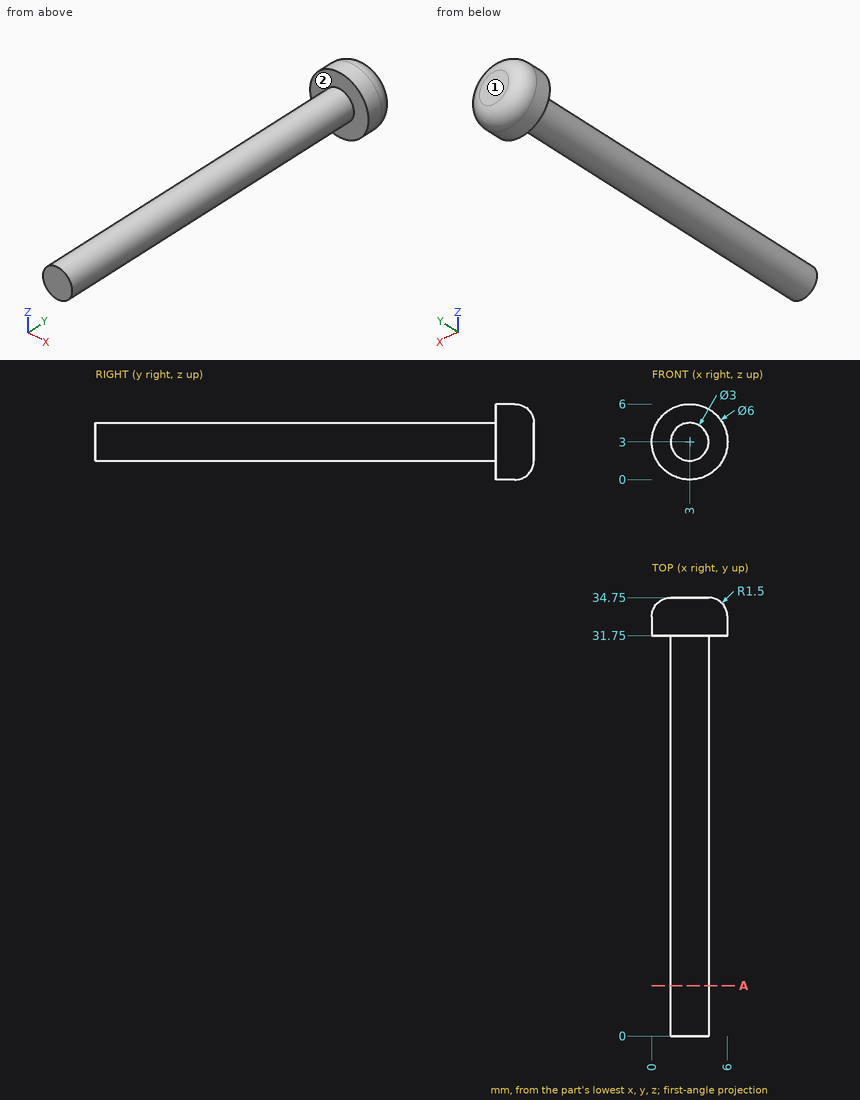
Job drawing, mm, ordinate dimensions from the low corner. One solid piece. A direction names the side the tool comes from. Coordinates: 2 decimals unless noted, no trailing zeros. Order: outer loops, then holes, each group sorted by start corner. A loop starts at its lowest first (then second) coordinate and runs counter-clockwise, first axis right, second up. Notation, with made-up numbers: (24, 35) - (30, 35) arc R23 cw to (30, 51) - close; hole circle Ø1 at (87.5, 53.5). An arc over 180 degrees is marked (long way). Write each question's results on one line, items separated by ' | '. Start each with the question number.
Item 1: Band-saw the part on A-A on y = 4. Write the cut outline in (x, z).
Item 2: Flat gauge pin, fed straight in: pin 1 (2 mm diameter, centred on x = 1, z = 3.5, fed in from +Y). Where does the tip first touch, or does it go through?
Item 3: Wall check: probe 1 along Y at (x, z) = (2.75, 4.65); probe 2 along Y at (x, z) = (0.75, 2.5); probe 3 along X at (y, z) = (24, 2.35). Give the ranges that are in metal, low to high. Write a range as [from, to].
Item 4: Tool access for the marked faces 1 and 2: list every direction of +Z, -Z, +X, -X, +Y, -Y with a clear straight run to the whole face (end or side of a thin tool).
Numbers:
1) outline: circle Ø3 at (3, 3)
2) pin 1: y = 34.75
3) probe 1: [31.75, 34.74] | probe 2: [31.75, 34.52] | probe 3: [1.65, 4.35]
4) face 1: +Z, -Z, +X, -X, +Y | face 2: -Y
